from build123d import *

# Parameters (mm, degrees)
F0_W          = 10
F0_H          = 15
F1_DEPTH      = 7
F3_DEPTH      = 60
F4_R          = 1.6
F5_DEPTH      = 60
F6_R          = 1.6
F7_DEPTH      = 60
F8_R          = 17.5
F9_DEPTH      = 25
F10_T1_DEPTH  = 35
F10_T3_DEPTH  = 35
F10_T5_DEPTH  = 35
F10_T7_DEPTH  = 35
F10_T9_DEPTH  = 35
F10_T11_DEPTH = 35


# Not quite as in the source:
# - a fillet or chamfer that OpenCascade refuses, or shapes differently, is made with other operations: its cross-section is extruded or revolved along the edge and cut away or added
# - a feature names something its author has since deleted; it is built from what else it names


with BuildPart() as f1:
    # F0 (on Top) → F1 (new body)
    with BuildSketch(Plane.XY):
        Polygon((-19.0935776077, -11.020506829), (-0.0410187244, -0.020506829), (-21.6916538191, 12.479493171), (-26.6916538191, 3.8192391331), (-31.6916538191, -4.8410149047), align=None)
        Polygon((-0.0410187244, 21.979493171), (-0.0410187244, -0.020506829), (21.6096163702, 12.479493171), (16.6096163702, 21.1397472088), (11.6096163702, 29.8000012467), align=None)
        Polygon((19.0115401588, -11.020506829), (-0.0410187244, -0.020506829), (-0.0410187244, -25.020506829), (9.9589812756, -25.020506829), (19.9589812756, -25.020506829), align=None)
        Polygon((-0.0410187244, -25.020506829), (-0.0410187244, -0.020506829), (-19.0935776077, -11.020506829), (-20.0410187244, -25.020506829), (-10.0410187244, -25.020506829), align=None)
        Polygon((-21.6916538191, 12.479493171), (-0.0410187244, -0.020506829), (-0.0410187244, 21.979493171), (-11.6916538191, 29.8000012467), (-16.6916538191, 21.1397472088), align=None)
        Polygon((21.6096163702, 12.479493171), (-0.0410187244, -0.020506829), (19.0115401588, -11.020506829), (31.6096163702, -4.8410149047), (26.6096163702, 3.8192391331), align=None)
        Polygon((-29.6820348758, 28.6397472088), (-16.6916538191, 21.1397472088), (-11.6916538191, 29.8000012467), (-24.6820348758, 37.3000012467), align=None)
        Polygon((-31.6916538191, -4.8410149047), (-26.6916538191, 3.8192391331), (-39.6820348758, 11.3192391331), (-44.6820348758, 2.6589850953), align=None)
        Polygon((39.5999974269, 11.3192391331), (26.6096163702, 3.8192391331), (31.6096163702, -4.8410149047), (44.5999974269, 2.6589850953), align=None)
        Polygon((11.6096163702, 29.8000012467), (16.6096163702, 21.1397472088), (29.5999974269, 28.6397472088), (24.5999974269, 37.3000012467), align=None)
        with Locations((-15.0410187244, -32.520506829)):
            Rectangle(F0_W, F0_H)
        with Locations((14.9589812756, -32.520506829)):
            Rectangle(F0_W, F0_H)
    extrude(amount=F1_DEPTH)

    # F2 (on face) → F3 (cut)
    with BuildSketch(Plane.YZ.offset(19.9589812756)):
        with BuildLine():
            ThreePointArc((-35.420506829, 3.5), (-37.020506829, 5.1), (-38.620506829, 3.5))
            ThreePointArc((-38.620506829, 3.5), (-37.020506829, 1.9), (-35.420506829, 3.5))
        make_face()
    extrude(amount=-F3_DEPTH, mode=Mode.SUBTRACT)

    # F4 (on face) → F5 (cut)
    with BuildSketch(Plane(origin=(9.9986250363, -17.3181265688, 0), x_dir=(0.8660254038, 0.5, 0), z_dir=(0.5, -0.8660254038, 0))):
        with Locations((36.9542233281, 3.5)):
            Circle(F4_R)
    extrude(amount=-F5_DEPTH, mode=Mode.SUBTRACT)

    # F6 (on face) → F7 (cut)
    with BuildSketch(Plane(origin=(9.9808656014, 17.2873663252, 0), x_dir=(-0.8660254038, 0.5, 0), z_dir=(0.5, 0.8660254038, 0))):
        with Locations((37.0252698429, 3.5)):
            Circle(F6_R)
    extrude(amount=-F7_DEPTH, mode=Mode.SUBTRACT)

    # F8 (on face) → F9 (cut)
    with BuildSketch(Plane.XY.offset(7)):
        Circle(F8_R)
    extrude(amount=-F9_DEPTH, mode=Mode.SUBTRACT)

    # F10: fillet of radius 5 on 12 edges, made by hand

    # F10_s2 → F10_t1 (cut)
    with BuildSketch(Plane.YZ.offset(-32.5410187244)):
        with BuildLine():
            ThreePointArc((-35.020506829, 7), (-38.556040735, 5.5355339059), (-40.020506829, 2))
            Line((-40.020506829, 2), (-40.020506829, 7))
            Line((-40.020506829, 7), (-35.020506829, 7))
        make_face()
        with BuildLine():
            ThreePointArc((-35.020506829, 0), (-38.556040735, 1.4644660941), (-40.020506829, 5))
            Line((-40.020506829, 5), (-40.020506829, 0))
            Line((-40.020506829, 0), (-35.020506829, 0))
        make_face()
    extrude(amount=F10_T1_DEPTH, mode=Mode.SUBTRACT)

    # F10_s4 → F10_t3 (cut)
    with BuildSketch(Plane.YZ.offset(-2.5410187244)):
        with BuildLine():
            ThreePointArc((-35.020506829, 0), (-38.556040735, 1.4644660941), (-40.020506829, 5))
            Line((-40.020506829, 5), (-40.020506829, 0))
            Line((-40.020506829, 0), (-35.020506829, 0))
        make_face()
        with BuildLine():
            ThreePointArc((-35.020506829, 7), (-38.556040735, 5.5355339059), (-40.020506829, 2))
            Line((-40.020506829, 2), (-40.020506829, 7))
            Line((-40.020506829, 7), (-35.020506829, 7))
        make_face()
    extrude(amount=F10_T3_DEPTH, mode=Mode.SUBTRACT)

    # F10_s6 → F10_t5 (cut)
    with BuildSketch(Plane(origin=(16.2486250363, -28.1434441161, 0), x_dir=(0, 0, 1), z_dir=(-0.5, 0.8660254038, 0))):
        with BuildLine():
            ThreePointArc((7, 34.9542233281), (5.5355339059, 38.489757234), (2, 39.9542233281))
            Line((2, 39.9542233281), (7, 39.9542233281))
            Line((7, 39.9542233281), (7, 34.9542233281))
        make_face()
        with BuildLine():
            ThreePointArc((0, 34.9542233281), (1.4644660941, 38.489757234), (5, 39.9542233281))
            Line((5, 39.9542233281), (0, 39.9542233281))
            Line((0, 39.9542233281), (0, 34.9542233281))
        make_face()
    extrude(amount=F10_T5_DEPTH, mode=Mode.SUBTRACT)

    # F10_s8 → F10_t7 (cut)
    with BuildSketch(Plane(origin=(1.2486250363, -2.1626820025, 0), x_dir=(0, 0, 1), z_dir=(-0.5, 0.8660254038, 0))):
        with BuildLine():
            ThreePointArc((7, 34.9542233281), (5.5355339059, 38.489757234), (2, 39.9542233281))
            Line((2, 39.9542233281), (7, 39.9542233281))
            Line((7, 39.9542233281), (7, 34.9542233281))
        make_face()
        with BuildLine():
            ThreePointArc((0, 34.9542233281), (1.4644660941, 38.489757234), (5, 39.9542233281))
            Line((5, 39.9542233281), (0, 39.9542233281))
            Line((0, 39.9542233281), (0, 34.9542233281))
        make_face()
    extrude(amount=F10_T7_DEPTH, mode=Mode.SUBTRACT)

    # F10_s10 → F10_t9 (cut)
    with BuildSketch(Plane(origin=(16.2308656014, 28.1126838725, 0), x_dir=(0, 0, 1), z_dir=(-0.5, -0.8660254038, 0))):
        with BuildLine():
            ThreePointArc((7, 35.0252698429), (5.5355339059, 38.5608037488), (2, 40.0252698429))
            Line((2, 40.0252698429), (7, 40.0252698429))
            Line((7, 40.0252698429), (7, 35.0252698429))
        make_face()
        with BuildLine():
            ThreePointArc((0, 35.0252698429), (1.4644660941, 38.5608037488), (5, 40.0252698429))
            Line((5, 40.0252698429), (0, 40.0252698429))
            Line((0, 40.0252698429), (0, 35.0252698429))
        make_face()
    extrude(amount=F10_T9_DEPTH, mode=Mode.SUBTRACT)

    # F10_s12 → F10_t11 (cut)
    with BuildSketch(Plane(origin=(1.2308656014, 2.131921759, 0), x_dir=(0, 0, 1), z_dir=(-0.5, -0.8660254038, 0))):
        with BuildLine():
            ThreePointArc((7, 35.0252698429), (5.5355339059, 38.5608037488), (2, 40.0252698429))
            Line((2, 40.0252698429), (7, 40.0252698429))
            Line((7, 40.0252698429), (7, 35.0252698429))
        make_face()
        with BuildLine():
            ThreePointArc((0, 35.0252698429), (1.4644660941, 38.5608037488), (5, 40.0252698429))
            Line((5, 40.0252698429), (0, 40.0252698429))
            Line((0, 40.0252698429), (0, 35.0252698429))
        make_face()
    extrude(amount=F10_T11_DEPTH, mode=Mode.SUBTRACT)


solid = f1.part
Geometry: final body of the model. Coordinates: model frame, mm. A direction names the side the tool comes from. Give positions to 0.01 mm unless a question says otherwise; leave off trailing zeros. Write each loop counter-clockwise with the first axis right and the second up, starting at its lowest first coordinate (ties: lowest second). Pieces come first, ordered by that corner, then holes.
(1) First-contact query: P1, Ø3.5, axis at y = -30.5, z = 5, coming from the +X side; P2, Ø3.5, axis at y = -28.5, z = 4.5, coming from the -X side; P3, Ø2, axis at y = -3, z = 2, coming from the +X side. Flat tips, straight axial feed; report the tip coordinate or a pass-through.
(2) Access query for faces 4 (the flat face through (16.67, 32.72, 3.45)), 5 (the flat face through (-10.041, -31, 3)), 6 (the flat face through (31.67, 6.74, 3.45)), 7 (the flat face through (19.959, -31, 3)). Directions: +Z, -Z, +X, -X, +Y, -Y. A direction counts if a zero-diameter tool reaches every point of the face in a straight line with its end or side. Return the directions, or none.
(3) Cut plane B-B, the plane y = 32. Give the number of separate pieces and of enclosed holes in the cut face, then the cut area to 3 significant figures.
(4) Cut plane A-A, the plane y = 16. Return loops of the section in (x, z).
(5) Mould query, pull axis Z, two halves, no side actions, for faces 1 (the cylindrical face through (-25.348, 31.992, 6.057)), 2 (the flat face through (-5.785, 25.835, 3.451)), 3 (the cylindrical face through (-38.45, 4.91, 2.53)). Classes: released by +Z, released by -Z, zero draft, split by the parting line, or undercut.
(6) Cut plane D-D, the plane x = 34. Return loops of the section in (y, z).
(7) Ray query, line 1 (X direction, y = -30, z = 5.5); line 2 (X direction, y = 9, z = 2.5) (1 decimal); line 3 (Y direction, x = 15, z = 3). Return the intervals inside material, ascending.
(8) Cut plane C-C, the plane y = -8.5. Return loops of the section in (x, z), then the cut area to 3 significant figures.
Values follow:
1. P1: stops at x = 19.96
1. P2: stops at x = -20.04
1. P3: stops at x = 36.53
2. face 4: +Z, -Z, +Y
2. face 5: +Z, -Z, -Y
2. face 6: +Z, -Z
2. face 7: +Z, -Z, +X, -Y
3. separate pieces: 2
3. enclosed holes: 2
3. area: 129 mm2
4. outline: (-19.66, 0) - (-7.09, 0) - (-7.09, 7) - (-19.66, 7) - close; (7.09, 0) - (19.58, 0) - (19.58, 7) - (7.09, 7) - close
5. face 1: released by +Z
5. face 2: zero draft
5. face 3: undercut
6. outline: (-3.46, 0) - (8.09, 0) - (8.09, 7) - (-3.46, 7) - close
7. line 1: x = -20.04 to -10.04, 9.96 to 19.96
7. line 2: x = -40.2 to -39, -36.1 to -35.7, -23.7 to -15, 15 to 23.6, 35.6 to 36, 38.9 to 40.2
7. line 3: y = -39.6 to -38.54, -35.5 to -9.01, 9.01 to 31.76
8. outline: (-24.23, 0) - (-15.3, 0) - (-15.3, 7) - (-24.23, 7) - close; (15.3, 0) - (24.15, 0) - (24.15, 7) - (15.3, 7) - close
8. area: 125 mm2
